from build123d import *

# Parameters (mm, degrees)
CYLINDER014_R          = 1.7
CYLINDER014_DEPTH      = 31
CYLINDER014_ROLL_ANGLE = 90
CYLINDER012_R          = 30
CYLINDER012_DEPTH      = 30
CYLINDER012_ROLL_ANGLE = 90
CYLINDER013_R          = 10
CYLINDER013_DEPTH      = 31
CYLINDER013_ROLL_ANGLE = 90
FILLET004_R            = 10
CYLINDER016_R          = 20
CYLINDER016_DEPTH      = 34
CYLINDER016_ROLL_ANGLE = 90
CYLINDER015_R          = 32
CYLINDER015_DEPTH      = 34
CYLINDER015_ROLL_ANGLE = 90
FILLET005_R            = 3


with BuildPart() as cilindro014:
    # Cylinder014 → Cylinder014 (new body)
    with BuildSketch(Plane.XY):
        Circle(CYLINDER014_R)
    extrude(amount=CYLINDER014_DEPTH)


with BuildPart() as cilindro014_1:
    # Cylinder014 roll: moved
    add(cilindro014.part.rotate(Axis((0, 0, 0), (1, 0, 0)), CYLINDER014_ROLL_ANGLE))


with BuildPart() as cilindro014_2:
    # Cylinder014 placement: moved
    add(cilindro014_1.part.moved(Location((220, 89, -34.5))))


with BuildPart() as cilindro012:
    # Cylinder012 → Cylinder012 (new body)
    with BuildSketch(Plane.XY):
        Circle(CYLINDER012_R)
    extrude(amount=CYLINDER012_DEPTH)


with BuildPart() as cilindro012_1:
    # Cylinder012 roll: moved
    add(cilindro012.part.rotate(Axis((0, 0, 0), (1, 0, 0)), CYLINDER012_ROLL_ANGLE))


with BuildPart() as cilindro012_2:
    # Cylinder012 placement: moved
    add(cilindro012_1.part.moved(Location((220, 89, -34.5))))


with BuildPart() as clone_of_fillet004:
    # Cylinder013 → Cylinder013 (new body)
    with BuildSketch(Plane.XY):
        Circle(CYLINDER013_R)
    extrude(amount=CYLINDER013_DEPTH)


with BuildPart() as clone_of_fillet004_1:
    # Cylinder013 roll: moved
    add(clone_of_fillet004.part.rotate(Axis((0, 0, 0), (1, 0, 0)), CYLINDER013_ROLL_ANGLE))


with BuildPart() as clone_of_fillet004_2:
    # Cylinder013 placement: moved
    add(clone_of_fillet004_1.part.moved(Location((220, 89, -34.5))))

    # Fusion015: union Cilindro012
    add(cilindro012_2.part)

    # Cut008: cut Cilindro014
    add(cilindro014_2.part, mode=Mode.SUBTRACT)

    # Fillet004
    fillet004_edges = [clone_of_fillet004_2.edges().sort_by_distance(p)[0] for p in [
        (190, 59, -34.5),
        (190, 89, -34.5),
    ]]
    fillet(fillet004_edges, radius=FILLET004_R)


with BuildPart() as cilindro016:
    # Cylinder016 → Cylinder016 (new body)
    with BuildSketch(Plane.XY):
        Circle(CYLINDER016_R)
    extrude(amount=CYLINDER016_DEPTH)


with BuildPart() as cilindro016_1:
    # Cylinder016 roll: moved
    add(cilindro016.part.rotate(Axis((0, 0, 0), (1, 0, 0)), CYLINDER016_ROLL_ANGLE))


with BuildPart() as cilindro016_2:
    # Cylinder016 placement: moved
    add(cilindro016_1.part.moved(Location((220, 91, -34.5))))


with BuildPart() as fillet005:
    # Cylinder015 → Cylinder015 (new body)
    with BuildSketch(Plane.XY):
        Circle(CYLINDER015_R)
    extrude(amount=CYLINDER015_DEPTH)


with BuildPart() as fillet005_1:
    # Cylinder015 roll: moved
    add(fillet005.part.rotate(Axis((0, 0, 0), (1, 0, 0)), CYLINDER015_ROLL_ANGLE))


with BuildPart() as fillet005_2:
    # Cylinder015 placement: moved
    add(fillet005_1.part.moved(Location((220, 91, -34.5))))

    # Cut009: cut Cilindro016
    add(cilindro016_2.part, mode=Mode.SUBTRACT)

    # Cut010: cut Clone of Fillet004
    add(clone_of_fillet004_2.part, mode=Mode.SUBTRACT)

    # Fillet005
    fillet005_edges = [fillet005_2.edges().sort_by_distance(p)[0] for p in [
        (188, 57, -34.5),
        (188, 91, -34.5),
    ]]
    fillet(fillet005_edges, radius=FILLET005_R)


with BuildPart() as part_mirroring002:
    # Part__Mirroring002: instance of Fillet005
    add(fillet005_2.part.mirror(Plane(origin=(0, 0, 0), x_dir=(1, 0, 0), z_dir=(0, 1, 0))))


solid = part_mirroring002.part
Here's how the part is built. I have some questions about the finished solid (model axes, mm). Round coordinates to 2 decimals unless told otherwise and drop trailing zeros. Write each loop counter-clockwise with the first axis right and the second up, starting at its lowest first coordinate (ties: lowest second). Pieces come first, ordered by that corner, then holes.
1. I need wall thicknesses on L1, parallel to Z at x = 220, y = -75; L2, parallel to X at y = -74, z = -34; L3, parallel to Y at x = 202, z = -55. Which ranges of each line are inside material? Lowest first, please.
2. Suppose I cut it at B-B (x = 220). List the corners of the cut face in (y, z) for me.
3. Will these pins go through, and if not, where does the flat tip stop? pin 1 Ø6 at (x, y) = (238.5, -73.5) entering from +Z; pin 2 Ø2 at (y, z) = (-65, -59) entering from +X; pin 3 Ø12 at (x, y) = (220, -65.5) entering from -Z.
4. Suppose I cut it at C-C (y = -72). List the corners of the cut face in (x, z) for me, and give its area (3 significant figures).
5. If we mould it in two halves opening along Z, with no side actions, what happens to faces 1 (the cylindrical face through (248.615, -74.07, -25.489)), 2 (the flat face through (200, -57, -41)), 3 (the cylindrical face through (205.26, -90.01, -20.98)), 4 (the cylindrical face through (194.606, -74.196, -53.972))? For each: released by +Z, released by -Z, zero draft, split by the parting line, or undercut.
6. Suppose I cut it at A-A (z = -34.5). List the corners of the cut face in (x, y) for me, and give its area (3 significant figures).
7. Suppose I cut it at D-D (y = -63). List the corners of the cut face in (x, z) for me.
Answer sheet:
1. L1: z = -66.5 to -64.5, -4.5 to -2.5
1. L2: x = 188 to 190, 250 to 252
1. L3: y = -91 to -85.85, -62.15 to -57
2. outline: (-91, -63.5) arc R3 ccw to (-88, -66.5) - (-60, -66.5) arc R3 ccw to (-57, -63.5) - (-57, -54.5) - (-59, -54.5) arc R10 cw to (-69, -64.5) - (-79, -64.5) arc R10 cw to (-89, -54.5) - (-91, -54.5) - close; (-91, -14.5) - (-89, -14.5) arc R10 cw to (-79, -4.5) - (-69, -4.5) arc R10 cw to (-59, -14.5) - (-57, -14.5) - (-57, -5.5) arc R3 ccw to (-60, -2.5) - (-88, -2.5) arc R3 ccw to (-91, -5.5) - close
3. pin 1: stops at z = -6.5
3. pin 2: stops at x = 241.72
3. pin 3: stops at z = -66.5
4. outline: circle Ø64 at (220, -34.5); hole circle Ø60 at (220, -34.5)
4. area: 390 mm2
5. face 1: undercut
5. face 2: zero draft
5. face 3: undercut
5. face 4: split by the parting line
6. outline: (188, -88) arc R3 ccw to (191, -91) - (200, -91) - (200, -89) arc R10 cw to (190, -79) - (190, -69) arc R10 cw to (200, -59) - (200, -57) - (191, -57) arc R3 ccw to (188, -60) - close; (240, -91) - (249, -91) arc R3 ccw to (252, -88) - (252, -60) arc R3 ccw to (249, -57) - (240, -57) - (240, -59) arc R10 cw to (250, -69) - (250, -79) arc R10 cw to (240, -89) - close
6. area: 294 mm2
7. outline: circle Ø64 at (220, -34.5); hole circle Ø56 at (220, -34.5)
